Geometry check sheet. Reference: the model listing, model coordinates, mm. A direction names the side the tool comes from. Give positions to 0.01 mm unless a question says otherwise; leave off trailing zeros. Order: outer loops, then holes, each group sorted by start corner. A loop starts at its lowest first (then second) coordinate and runs counter-clockwise, first axis right, second up. Notation, with made-up numbers: M 42,11.25 L 95,11.25 A18 ccw 95,15.25 Z; hole C -23.75,-19.75 d5. An arc over 180 degrees is marked long. Put each result on its own line as item: value. Start each with the question number.
Q1. Material ranges on L1, parallel to Z at x = 0, y = -1.25; L2, parallel to X at y = -2.75, z = -9.5; L3, parallel to Z at x = 0, y = -4, recorded low to high.
Q2. Mould release check, pull along Z, two halves, no side actions. Record for faces 1 (the flat face through (-9.36, -3.94, 19.79)), 2 (the cylindrical face through (-21.838, -4.766, -0.165)), 3 (the cylindrical face through (-5.128, -4.958, -22.854)): +Z half, -Z half, draft (parallel to the pull), parting line (faces both ways), or undercut.
Q3. Access from +Z, -Z, +X, -X, +Y, -Y to the whole of each face (thin tool, end or side, straight path). Record for faces 4 (the cylindrical face through (0.074, -4.958, -19.603)), 5 (the cylindrical face through (-0.43, -3.94, 22.33)), 6 (the flat face through (-17.6, -3.9, 11.75)), 7 (the flat face through (-17.7, -3.9, -11.75)).
Q4. Go/stop test with flat-tipped pins: pin 1 (3 mm diameter, centred on x = -10.5, y = -5.5, fed in from -Z); pin 2 (1.5 mm diameter, centred on x = 10.5, y = -4.5, fed in from +Z); pin 3 (8.5 mm diameter, centred on x = 5, z = 5, fed in from -Y). Record where each tip stops, or that it passes through.
Q5. Section check B-B on y = -4.75. State how many separate pieces and enclosed holes the cut face has, then the cut area to 3 significant figures.
Q6. Section check A-A on x = 0. Record the cut outline in (y, z), then the cut area to 3 significant figures.
Q7. Section check D-D on y = -1. Record the cut outline in (x, z), then the cut area to 3 significant figures.
Q8. Section check C-C on z = 1.5. Record the cut outline in (x, y).
```python
from build123d import *

# Parameters (mm, degrees)
F0_R     = 2
F1_DEPTH = 8
F2_DEPTH = 2
F3_R     = 1
F5_D     = 4
F6_R     = 4


# Not quite as in the source:
# - a feature names something its author has since deleted; it is built from what else it names


with BuildPart() as f1:
    # F0 (on Front) → F1 (new body)
    with BuildSketch(Plane.XZ):
        with BuildLine():
            Line((15.1970139668, 6.8636525628), (6.0880650012, 27.0320429916))
            ThreePointArc((6.0880650012, 27.0320429916), (0, 30.9626), (-6.0880650012, 27.0320429916))
            Line((-6.0880650012, 27.0320429916), (-12.9901204821, 11.75))
            Line((-12.9901204821, 11.75), (-12.9901204821, 6.8910419314))
            Line((-12.9901204821, 6.8910419314), (-6.0462846285, 22.2655920687))
            ThreePointArc((-6.0462846285, 22.2655920687), (-5.1436901116, 22.8539427752), (-4.2309206889, 22.2815046593))
            ThreePointArc((-4.2309206889, 22.2815046593), (0, 19.6022), (4.2309206889, 22.2815046593))
            ThreePointArc((4.2309206889, 22.2815046593), (5.1436901116, 22.8539427752), (6.0462846285, 22.2655920687))
            Line((6.0462846285, 22.2655920687), (13.3742945868, 6.0404308054))
            ThreePointArc((13.3742945868, 6.0404308054), (14.6751, 0), (13.3742945868, -6.0404308054))
            Line((13.3742945868, -6.0404308054), (6.0462846285, -22.2655920687))
            ThreePointArc((6.0462846285, -22.2655920687), (5.1436901116, -22.8539427752), (4.2309206889, -22.2815046593))
            ThreePointArc((4.2309206889, -22.2815046593), (0, -19.6022), (-4.2309206889, -22.2815046593))
            ThreePointArc((-4.2309206889, -22.2815046593), (-5.1436901116, -22.8539427752), (-6.0462846285, -22.2655920687))
            Line((-6.0462846285, -22.2655920687), (-12.9901204821, -6.8910419314))
            Line((-12.9901204821, -6.8910419314), (-12.9901204821, -11.75))
            Line((-12.9901204821, -11.75), (-6.0880650012, -27.0320429916))
            ThreePointArc((-6.0880650012, -27.0320429916), (0, -30.9626), (6.0880650012, -27.0320429916))
            Line((6.0880650012, -27.0320429916), (15.1970139668, -6.8636525628))
            ThreePointArc((15.1970139668, -6.8636525628), (16.6751, 0), (15.1970139668, 6.8636525628))
        make_face()
        with Locations((0, -24.2824)):
            Circle(F0_R, mode=Mode.SUBTRACT)
        with Locations((0, 24.2824)):
            Circle(F0_R, mode=Mode.SUBTRACT)
        Polygon((-12.9901204821, 6.8910419314), (-12.9901204821, 11.75), (-23.9901204821, 11.75), (-23.9901204821, -11.75), (-12.9901204821, -11.75), (-12.9901204821, -6.8910419314), align=None)
    extrude(amount=F1_DEPTH)

    # F0 (on Front) → F2 (join)
    with BuildSketch(Plane.XZ):
        with BuildLine():
            Line((-6.0462846285, 22.2655920687), (-12.9901204821, 6.8910419314))
            Line((-12.9901204821, 6.8910419314), (-12.9901204821, -6.8910419314))
            Line((-12.9901204821, -6.8910419314), (-6.0462846285, -22.2655920687))
            ThreePointArc((-6.0462846285, -22.2655920687), (-5.1436901116, -22.8539427752), (-4.2309206889, -22.2815046593))
            ThreePointArc((-4.2309206889, -22.2815046593), (0, -19.6022), (4.2309206889, -22.2815046593))
            ThreePointArc((4.2309206889, -22.2815046593), (5.1436901116, -22.8539427752), (6.0462846285, -22.2655920687))
            Line((6.0462846285, -22.2655920687), (13.3742945868, -6.0404308054))
            ThreePointArc((13.3742945868, -6.0404308054), (14.6751, 0), (13.3742945868, 6.0404308054))
            Line((13.3742945868, 6.0404308054), (6.0462846285, 22.2655920687))
            ThreePointArc((6.0462846285, 22.2655920687), (5.1436901116, 22.8539427752), (4.2309206889, 22.2815046593))
            ThreePointArc((4.2309206889, 22.2815046593), (0, 19.6022), (-4.2309206889, 22.2815046593))
            ThreePointArc((-4.2309206889, 22.2815046593), (-5.1436901116, 22.8539427752), (-6.0462846285, 22.2655920687))
        make_face()
        Polygon((-12.9901204821, 6.8910419314), (-12.9901204821, 11.75), (-23.9901204821, 11.75), (-23.9901204821, -11.75), (-12.9901204821, -11.75), (-12.9901204821, -6.8910419314), align=None)
        with BuildLine():
            Line((15.1970139668, 6.8636525628), (6.0880650012, 27.0320429916))
            ThreePointArc((6.0880650012, 27.0320429916), (0, 30.9626), (-6.0880650012, 27.0320429916))
            Line((-6.0880650012, 27.0320429916), (-12.9901204821, 11.75))
            Line((-12.9901204821, 11.75), (-12.9901204821, 6.8910419314))
            Line((-12.9901204821, 6.8910419314), (-6.0462846285, 22.2655920687))
            ThreePointArc((-6.0462846285, 22.2655920687), (-5.1436901116, 22.8539427752), (-4.2309206889, 22.2815046593))
            ThreePointArc((-4.2309206889, 22.2815046593), (0, 19.6022), (4.2309206889, 22.2815046593))
            ThreePointArc((4.2309206889, 22.2815046593), (5.1436901116, 22.8539427752), (6.0462846285, 22.2655920687))
            Line((6.0462846285, 22.2655920687), (13.3742945868, 6.0404308054))
            ThreePointArc((13.3742945868, 6.0404308054), (14.6751, 0), (13.3742945868, -6.0404308054))
            Line((13.3742945868, -6.0404308054), (6.0462846285, -22.2655920687))
            ThreePointArc((6.0462846285, -22.2655920687), (5.1436901116, -22.8539427752), (4.2309206889, -22.2815046593))
            ThreePointArc((4.2309206889, -22.2815046593), (0, -19.6022), (-4.2309206889, -22.2815046593))
            ThreePointArc((-4.2309206889, -22.2815046593), (-5.1436901116, -22.8539427752), (-6.0462846285, -22.2655920687))
            Line((-6.0462846285, -22.2655920687), (-12.9901204821, -6.8910419314))
            Line((-12.9901204821, -6.8910419314), (-12.9901204821, -11.75))
            Line((-12.9901204821, -11.75), (-6.0880650012, -27.0320429916))
            ThreePointArc((-6.0880650012, -27.0320429916), (0, -30.9626), (6.0880650012, -27.0320429916))
            Line((6.0880650012, -27.0320429916), (15.1970139668, -6.8636525628))
            ThreePointArc((15.1970139668, -6.8636525628), (16.6751, 0), (15.1970139668, 6.8636525628))
        make_face()
        with Locations((0, -24.2824)):
            Circle(F0_R, mode=Mode.SUBTRACT)
        with Locations((0, 24.2824)):
            Circle(F0_R, mode=Mode.SUBTRACT)
    extrude(amount=F2_DEPTH)

    # F3
    f3_edges = [f1.edges().sort_by_distance(p)[0] for p in [
        (-12.99012, -4, -11.75),
        (-12.99012, -4, 11.75),
    ]]
    fillet(f3_edges, radius=F3_R)

    # F5 (through all)
    with Locations(Plane.XY.offset(11.75)):
        with Locations((-19.9901204821, -4)):
            Hole(F5_D / 2)

    # F6
    f6_edges = [f1.edges().sort_by_distance(p)[0] for p in [
        (-23.99012, -8, 0),
    ]]
    fillet(f6_edges, radius=F6_R)


solid = f1.part
```
Results found:
1. L1: z = -30.96 to -26.28, -22.28 to 22.28, 26.28 to 30.96
1. L2: x = -23.99 to -21.55, -18.43 to -11.81, 11.81 to 14.01
1. L3: z = -30.96 to -26.28, -22.28 to -19.6, 19.6 to 22.28, 26.28 to 30.96
2. face 1: +Z half
2. face 2: draft
2. face 3: undercut
3. face 4: -Y
3. face 5: +Y, -Y
3. face 6: +Z, -X, +Y, -Y
3. face 7: -Z, -X, +Y, -Y
4. pin 1: stops at z = -20.58
4. pin 2: stops at z = 18.92
4. pin 3: stops at y = -2
5. separate pieces: 2
5. enclosed holes: 3
5. area: 532 mm^2
6. outline: M -8,-30.96 L 0,-30.96 L 0,-26.28 L -8,-26.28 Z; M -8,-22.28 L 0,-22.28 L 0,22.28 L -8,22.28 L -8,19.6 L -2,19.6 L -2,-19.6 L -8,-19.6 Z; M -8,26.28 L 0,26.28 L 0,30.96 L -8,30.96 Z
6. area: 196 mm^2
7. outline: M -23.99,-11.75 L -13.64,-11.75 A1 cw -12.72,-12.34 L -6.09,-27.03 A6.68 ccw 6.09,-27.03 L 15.2,-6.86 A16.68 ccw 15.2,6.86 L 6.09,27.03 A6.68 ccw -6.09,27.03 L -12.72,12.34 A1 cw -13.64,11.75 L -23.99,11.75 Z; hole C 0,-24.28 d4; hole C 0,24.28 d4
7. area: 1,550 mm^2
8. outline: M -23.99,-4 A4 ccw -19.99,-8 L -12.99,-8 L -12.99,-2 L 14.6,-2 L 14.6,-8 L 16.61,-8 L 16.61,0 L -23.99,0 Z; hole C -19.99,-4 d4
